Could you check a few things on this drawing? It's one solid part, dimensions in mm from its lowest x, y, z. A direction names the side the tool comes from. Give positions to 0.01 mm unless a question says otherwise; leave off trailing zeros. Order: outer loops, then holes, each group sorted by start corner. A loop starts at its lowest first (then second) coordinate and runs counter-clockwise, first axis right, second up. Notation, with made-up numbers: (40, -9) -> (54, -9) arc R32 ccw to (54, 18) -> close; hole circle Ø3 at (-23, 66.25). An arc over 180 degrees is marked (long way). Answer as a JSON object with one key per item and string values.
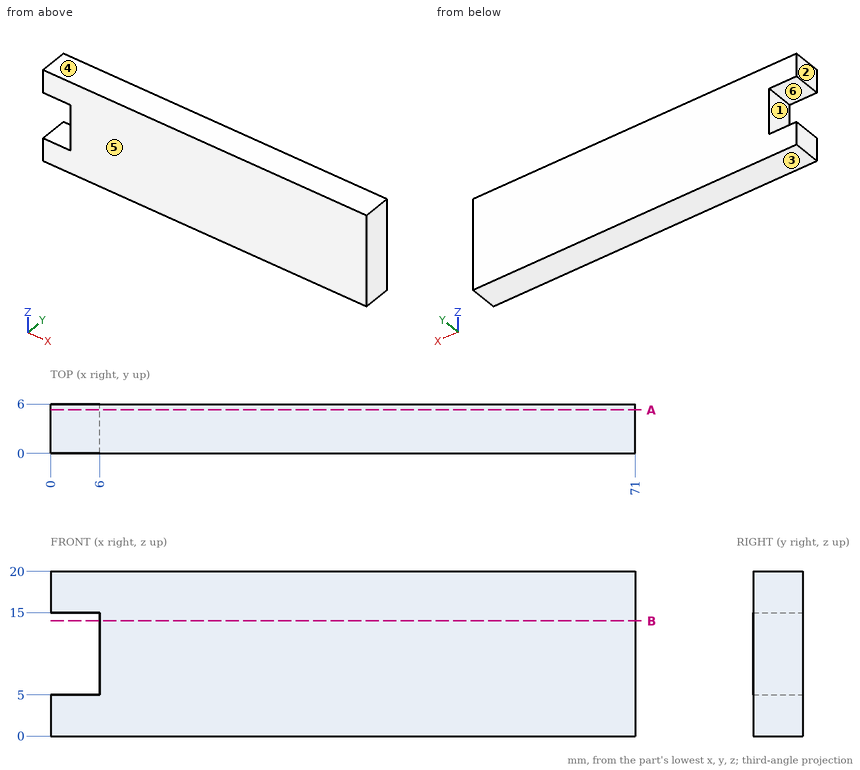
1. If we section it at A-A on y = 5.3: Please give me the cut outline in (x, z), then the cut area to 3 significant figures.
Worked answers:
{"outline": "(0, 0) -> (71, 0) -> (71, 20) -> (0, 20) -> (0, 15) -> (6, 15) -> (6, 5) -> (0, 5) -> close", "area": "1,360 mm²"}
2. Please list where these lines run through material, in increasing order: L1, parallel to Z at x = 3.5, y = 2.15; L2, parallel to X at y = 3, z = 12.25.
Worked answers:
{"L1": "0 to 5, 15 to 20", "L2": "6 to 71"}
3. If we section it at B-B on z = 14: Please give me the cut outline in (x, y).
Worked answers:
{"outline": "(6, 0) -> (71, 0) -> (71, 6) -> (6, 6) -> close"}
4. For the marked faces 5 and 6, which set-ups out of +Z, -Z, +X, -X, +Y, -Y let a thin tool reach every point of the face, with its end or its side?
Worked answers:
{"face 5": "+Z, -Z, +X, -X, -Y", "face 6": "-X, +Y, -Y"}
5. If we mould it in two halves opening along Z, with no side actions, what happens to the marked faces 1, 2, 3 and 4? For each: +Z half, -Z half, draft (parallel to the pull), parting line (faces both ways), or undercut.
Worked answers:
{"face 1": "undercut", "face 2": "draft", "face 3": "-Z half", "face 4": "+Z half"}
